from build123d import *

# Parameters (mm, degrees)
F1_DEPTH = 7.8
F3_DEPTH = 6.2
F4_DEPTH = 1.6
F6_DEPTH = 8
F8_DEPTH = 8.7


with BuildPart() as f1:
    # F0 (on Top) → F1 (new body)
    with BuildSketch(Plane.XY):
        with BuildLine():
            ThreePointArc((0, -3.5), (2.4748737342, -2.4748737342), (3.5, 0))
            Line((3.5, 0), (0, 0))
            Line((0, 0), (0, -3.5))
        make_face()
        with BuildLine():
            Line((0, 0), (3.5, 0))
            ThreePointArc((3.5, 0), (1.7904958486, 3.0073451109), (-1.6680712092, 3.0769365351))
            Line((-1.6680712092, 3.0769365351), (-0.7059061386, 1.9302728555))
            Line((-0.7059061386, 1.9302728555), (-1.2421372488, 1.4803215287))
            Line((-1.2421372488, 1.4803215287), (-1.778368359, 1.030370202))
            Line((-1.778368359, 1.030370202), (-2.7405334296, 2.1770338815))
            ThreePointArc((-2.7405334296, 2.1770338815), (-3.1519532504, -1.5215750745), (0, -3.5))
            Line((0, -3.5), (0, 0))
        make_face()
    extrude(amount=F1_DEPTH)

    # F2 (on face) → F3 (cut)
    with BuildSketch(Plane.XY.offset(7.8)):
        with BuildLine():
            ThreePointArc((-2.0789213734, 1.3885553367), (-0.7254986445, -2.3924154566), (2.5, 0))
            ThreePointArc((2.5, 0), (1.3663550266, 2.0935792178), (-1.0064591531, 2.2884579903))
            Line((-1.0064591531, 2.2884579903), (-0.7059061386, 1.9302728555))
            Line((-0.7059061386, 1.9302728555), (-1.778368359, 1.030370202))
            Line((-1.778368359, 1.030370202), (-2.0789213734, 1.3885553367))
        make_face()
    extrude(amount=-F3_DEPTH, mode=Mode.SUBTRACT)

    # F0 (on Top) → F4 (join)
    with BuildSketch(Plane.XY):
        with BuildLine():
            Line((-0.7059061386, 1.9302728555), (-1.6680712092, 3.0769365351))
            ThreePointArc((-1.6680712092, 3.0769365351), (-2.2497566339, 2.6811555509), (-2.7405334296, 2.1770338815))
            Line((-2.7405334296, 2.1770338815), (-1.778368359, 1.030370202))
            Line((-1.778368359, 1.030370202), (-1.2421372488, 1.4803215287))
            Line((-1.2421372488, 1.4803215287), (-0.7059061386, 1.9302728555))
        make_face()
        with BuildLine():
            Line((4.5, 0), (3.5, 0))
            ThreePointArc((3.5, 0), (2.4748737342, -2.4748737342), (0, -3.5))
            Line((0, -3.5), (0, -4.5))
            ThreePointArc((0, -4.5), (3.1819805153, -3.1819805153), (4.5, 0))
        make_face()
    extrude(amount=F4_DEPTH)

    # F5 (on face) → F6 (join)
    with BuildSketch(Plane(origin=(0, 0, 0), x_dir=(1, 0, 0), z_dir=(0, 0, -1))):
        Polygon((-2.1566756826, 0), (0, -2.1566756826), (2.1566756826, 0), (0, 2.1566756826), align=None)
    extrude(amount=F6_DEPTH)

    # F7 (on face) → F8 (join)
    with BuildSketch(Plane(origin=(0, 0, -8), x_dir=(1, 0, 0), z_dir=(0, 0, -1))):
        with BuildLine():
            Line((0, -2.1566756826), (-2.1566756826, 0))
            ThreePointArc((-2.1566756826, 0), (-1.525, -1.525), (0, -2.1566756826))
        make_face()
        with BuildLine():
            ThreePointArc((2.1566756826, 0), (1.525, 1.525), (0, 2.1566756826))
            Line((0, 2.1566756826), (2.1566756826, 0))
        make_face()
    extrude(amount=-F8_DEPTH)


solid = f1.part
Part model, mm, in its own coordinate system. A direction names the side the tool comes from. Coordinates: 2 decimals unless noted, no trailing zeros. Order: outer loops, then holes, each group sorted by start corner. A loop starts at its lowest first (then second) coordinate and runs counter-clockwise, first axis right, second up.
(1) Slice it at D-D, the plane z = 1. Write the cut outline in (x, y).
Check sheet entries:
outline: (0, -4.5) arc R4.5 ccw to (4.5, 0) - (3.5, 0) arc R3.5 ccw (long way) to (0, -3.5) - close
(2) Probe L1, parallel to Y at x = 0, z = 5.25; L2, parallel to Z at x = -2.5, y = -1. List the from-to ranges inside material, lowest first.
Check sheet entries:
L1: y = -3.5 to -2.5, 2.5 to 3.5
L2: z = 0 to 7.8
(3) Pin check, flat tips, straight feed: pin 1 Ø2 at (y, z) = (1.5, 5.5) entering from -X; pin 2 Ø3 at (x, z) = (-1, 0.5) entering from -Y; pin 3 Ø1 at (x, y) = (1, 0) entering from +Z; pin 4 Ø3 at (x, z) = (-2.5, 5) entering from -Y. Stop position of each tip, or through.
Check sheet entries:
pin 1: stops at x = -3.46
pin 2: stops at y = -4.5
pin 3: stops at z = 1.6
pin 4: stops at y = -3.35
(4) Slice it at C-C, the plane y = -3.25. Write the cut outline in (x, z).
Check sheet entries:
outline: (-1.3, 0) - (3.11, 0) - (3.11, 1.6) - (1.3, 1.6) - (1.3, 7.8) - (-1.3, 7.8) - close
(5) Slice it at A-A, the plane z = 6.25. Write the cut outline in (x, y).
Check sheet entries:
outline: (-2.74, 2.18) arc R3.5 ccw (long way) to (-1.67, 3.08) - (-1.01, 2.29) arc R2.5 cw (long way) to (-2.08, 1.39) - close
(6) Slice it at B-B, the plane x = -0.75. Write the cut outline in (y, z), and give its area (3 significant figures).
Check sheet entries:
outline: (-3.42, 0) - (-1.41, 0) - (-1.41, -8) - (2.02, -8) - (2.02, 0) - (3.42, 0) - (3.42, 7.8) - (2.38, 7.8) - (2.38, 1.6) - (-2.38, 1.6) - (-2.38, 7.8) - (-3.42, 7.8) - close
area: 51.2 mm2
(7) Tool access for faces 4 (the face through (1.063, 1.093, -3.944)), 5 (the face through (1.3, 1.3, 0)), 6 (the face through (0, -4, 1)), 7 (the face through (3, -3, 1.6)): list every direction of +Z, -Z, +X, -X, +Y, -Y with a clear straight run to the whole face (end or side of a thin tool).
Check sheet entries:
face 4: -Z, +X, +Y
face 5: -Z
face 6: +Z, -Z, -X, -Y
face 7: +Z, +X, -Y
(8) Pull direction X, two halves, no side cores. Call faces 1 (the face through (-1.063, -1.093, -3.944)), 2 (the face through (3.147, -3.217, 0.789)), 3 (the face through (0, 0, 1.6)): pulls with the +X half, pulls with the -X half, needs draft (parallel to the pull), parting line crosses it, or undercut.
Check sheet entries:
face 1: pulls with the -X half
face 2: pulls with the +X half
face 3: undercut
